Work out the finished part from the listing and answer in its coordinate system (mm). Face numbers are marked on the shaded views. Round coordinates to 2 decimals unless told otherwise and drop trailing zeros. Order: outer loops, then holes, each group sorted by start corner. A loop starts at its lowest first (then second) coordinate and runs counter-clockwise, first axis right, second up. Notation, with made-up numbers: (21, -16) - (27, -16) arc R19 ccw to (27, 10) - close; hole circle Ø1 at (-33, 22.25). An arc over 180 degrees is marked (long way). Answer in a Markdown table with one row per item.
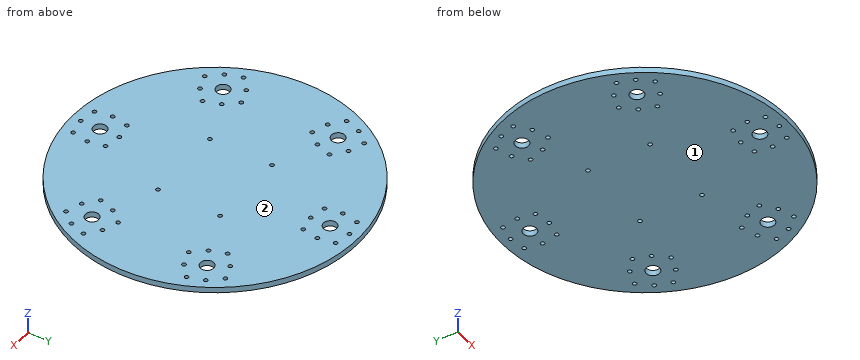
from build123d import *

# Parameters (mm, degrees)
SKETCH1_R           = 80
SKETCH1_R_2         = 1.1
SKETCH1_R_3         = 3.7
SKETCH1_R_4         = 1.11125
BOSS_EXTRUDE2_DEPTH = 3.175


with BuildPart() as part:
    # Sketch1 → Boss-Extrude2 (new body)
    with BuildSketch(Plane.XY):
        Circle(SKETCH1_R)
        with Locations((58.725568667, 44.315554285)):
            Circle(SKETCH1_R_2, mode=Mode.SUBTRACT)
        with Locations((67.741180127, 28.700057175)):
            Circle(SKETCH1_R_2, mode=Mode.SUBTRACT)
        with Locations((64.735398933, 37.375)):
            Circle(SKETCH1_R_2, mode=Mode.SUBTRACT)
        with Locations((50.050625842, 41.309773091)):
            Circle(SKETCH1_R_2, mode=Mode.SUBTRACT)
        with Locations((52.125683017, 19.684445715)):
            Circle(SKETCH1_R_2, mode=Mode.SUBTRACT)
        with Locations((43.110071557, 35.299942825)):
            Circle(SKETCH1_R_2, mode=Mode.SUBTRACT)
        with Locations((60.800625842, 22.690226909)):
            Circle(SKETCH1_R_2, mode=Mode.SUBTRACT)
        with Locations((46.115852752, 26.625)):
            Circle(SKETCH1_R_2, mode=Mode.SUBTRACT)
        with Locations((55.425625842, 32)):
            Circle(SKETCH1_R_3, mode=Mode.SUBTRACT)
        with Locations((-10.75, 64)):
            Circle(SKETCH1_R_2, mode=Mode.SUBTRACT)
        with Locations((-9.01561146, 73.01561146)):
            Circle(SKETCH1_R_2, mode=Mode.SUBTRACT)
        with Locations((9.01561146, 73.01561146)):
            Circle(SKETCH1_R_2, mode=Mode.SUBTRACT)
        with Locations((9.01561146, 54.98438854)):
            Circle(SKETCH1_R_2, mode=Mode.SUBTRACT)
        with Locations((-9.01561146, 54.98438854)):
            Circle(SKETCH1_R_2, mode=Mode.SUBTRACT)
        with Locations((0, 74.75)):
            Circle(SKETCH1_R_2, mode=Mode.SUBTRACT)
        with Locations((10.75, 64)):
            Circle(SKETCH1_R_2, mode=Mode.SUBTRACT)
        with Locations((0, 53.25)):
            Circle(SKETCH1_R_2, mode=Mode.SUBTRACT)
        with Locations((0, 64)):
            Circle(SKETCH1_R_3, mode=Mode.SUBTRACT)
        with Locations((67.741180127, -28.700057175)):
            Circle(SKETCH1_R_2, mode=Mode.SUBTRACT)
        with Locations((58.725568667, -44.315554285)):
            Circle(SKETCH1_R_2, mode=Mode.SUBTRACT)
        with Locations((64.735398933, -37.375)):
            Circle(SKETCH1_R_2, mode=Mode.SUBTRACT)
        with Locations((60.800625842, -22.690226909)):
            Circle(SKETCH1_R_2, mode=Mode.SUBTRACT)
        with Locations((43.110071557, -35.299942825)):
            Circle(SKETCH1_R_2, mode=Mode.SUBTRACT)
        with Locations((52.125683017, -19.684445715)):
            Circle(SKETCH1_R_2, mode=Mode.SUBTRACT)
        with Locations((50.050625842, -41.309773091)):
            Circle(SKETCH1_R_2, mode=Mode.SUBTRACT)
        with Locations((46.115852752, -26.625)):
            Circle(SKETCH1_R_2, mode=Mode.SUBTRACT)
        with Locations((55.425625842, -32)):
            Circle(SKETCH1_R_3, mode=Mode.SUBTRACT)
        with Locations((9.01561146, -73.01561146)):
            Circle(SKETCH1_R_2, mode=Mode.SUBTRACT)
        with Locations((-9.01561146, -73.01561146)):
            Circle(SKETCH1_R_2, mode=Mode.SUBTRACT)
        with Locations((0, -74.75)):
            Circle(SKETCH1_R_2, mode=Mode.SUBTRACT)
        with Locations((10.75, -64)):
            Circle(SKETCH1_R_2, mode=Mode.SUBTRACT)
        with Locations((-9.01561146, -54.98438854)):
            Circle(SKETCH1_R_2, mode=Mode.SUBTRACT)
        with Locations((9.01561146, -54.98438854)):
            Circle(SKETCH1_R_2, mode=Mode.SUBTRACT)
        with Locations((-10.75, -64)):
            Circle(SKETCH1_R_2, mode=Mode.SUBTRACT)
        with Locations((0, -53.25)):
            Circle(SKETCH1_R_2, mode=Mode.SUBTRACT)
        with Locations((0, -64)):
            Circle(SKETCH1_R_3, mode=Mode.SUBTRACT)
        with Locations((-58.725568667, -44.315554285)):
            Circle(SKETCH1_R_2, mode=Mode.SUBTRACT)
        with Locations((-67.741180127, -28.700057175)):
            Circle(SKETCH1_R_2, mode=Mode.SUBTRACT)
        with Locations((-64.735398933, -37.375)):
            Circle(SKETCH1_R_2, mode=Mode.SUBTRACT)
        with Locations((-50.050625842, -41.309773091)):
            Circle(SKETCH1_R_2, mode=Mode.SUBTRACT)
        with Locations((-52.125683017, -19.684445715)):
            Circle(SKETCH1_R_2, mode=Mode.SUBTRACT)
        with Locations((-43.110071557, -35.299942825)):
            Circle(SKETCH1_R_2, mode=Mode.SUBTRACT)
        with Locations((-60.800625842, -22.690226909)):
            Circle(SKETCH1_R_2, mode=Mode.SUBTRACT)
        with Locations((-46.115852752, -26.625)):
            Circle(SKETCH1_R_2, mode=Mode.SUBTRACT)
        with Locations((-55.425625842, -32)):
            Circle(SKETCH1_R_3, mode=Mode.SUBTRACT)
        with Locations((-67.741180127, 28.700057175)):
            Circle(SKETCH1_R_2, mode=Mode.SUBTRACT)
        with Locations((-58.725568667, 44.315554285)):
            Circle(SKETCH1_R_2, mode=Mode.SUBTRACT)
        with Locations((-64.735398933, 37.375)):
            Circle(SKETCH1_R_2, mode=Mode.SUBTRACT)
        with Locations((-60.800625842, 22.690226909)):
            Circle(SKETCH1_R_2, mode=Mode.SUBTRACT)
        with Locations((-43.110071557, 35.299942825)):
            Circle(SKETCH1_R_2, mode=Mode.SUBTRACT)
        with Locations((-52.125683017, 19.684445715)):
            Circle(SKETCH1_R_2, mode=Mode.SUBTRACT)
        with Locations((-50.050625842, 41.309773091)):
            Circle(SKETCH1_R_2, mode=Mode.SUBTRACT)
        with Locations((-46.115852752, 26.625)):
            Circle(SKETCH1_R_2, mode=Mode.SUBTRACT)
        with Locations((-55.425625842, 32)):
            Circle(SKETCH1_R_3, mode=Mode.SUBTRACT)
        with Locations((22.0345, 17.272)):
            Circle(SKETCH1_R_4, mode=Mode.SUBTRACT)
        with Locations((22.0345, -17.272)):
            Circle(SKETCH1_R_4, mode=Mode.SUBTRACT)
        with Locations((-21.9075, -17.272)):
            Circle(SKETCH1_R_4, mode=Mode.SUBTRACT)
        with Locations((-21.9075, 17.272)):
            Circle(SKETCH1_R_4, mode=Mode.SUBTRACT)
    extrude(amount=BOSS_EXTRUDE2_DEPTH)


solid = part.part
1) Find section C-C, the plane x = -27. Give the vertices of the cut face in (y, z) (3 decimals), then the cut area to 3 significant figures.
Filled in:
| item | result |
|---|---|
| outline | (-75.306, 0) - (75.306, 0) - (75.306, 3.175) - (-75.306, 3.175) - close |
| area | 478 mm^2 |
2) This flat-tipped pin is pushed along its axis until it touches: pin 1 (1 mm diameter, centred on y = -21, z = 2, fed in from +X). Where does it stop, or does it pass through?
Filled in:
| item | result |
|---|---|
| pin 1 | stops at x = 77.33 |
3) Find the intervals of material crossed by probe 1 along X at (y, z) = (54.5, 0.35); probe 2 along X at (y, z) = (-55.5, 0.7); probe 3 along Y at (x, z) = (-9.5, 0.9), in increasing order. Write a range as from..to.
Filled in:
| item | result |
|---|---|
| probe 1 | x = -58.56..-10, -8.03..8.03, 10..58.56 |
| probe 2 | x = -57.62..-9.99, -8.04..8.04, 9.99..57.62 |
| probe 3 | y = -79.43..-74, -72.03..-55.97, -54..54, 55.97..72.03, 74..79.43 |
4) The mould has two halves that part along Z. Classify the marked faces 1 and 2: released by +Z, released by -Z, zero draft, split by the parting line, or undercut.
Filled in:
| item | result |
|---|---|
| face 1 | released by -Z |
| face 2 | released by +Z |
5) Find section B-B, the plane z = 1.2. Give the number of separate pieces and of enclosed holes in the cut face, then the cut area to 3 significant figures.
Filled in:
| item | result |
|---|---|
| separate pieces | 1 |
| enclosed holes | 58 |
| area | 19,700 mm^2 |
6) Find section A-A, the plane y = -32. Give the vertices of the cut face in (x, z) (3 decimals).
Filled in:
| item | result |
|---|---|
| outline | (-73.321, 0) - (-59.126, 0) - (-59.126, 3.175) - (-73.321, 3.175) - close; (-51.726, 0) - (51.726, 0) - (51.726, 3.175) - (-51.726, 3.175) - close; (59.126, 0) - (73.321, 0) - (73.321, 3.175) - (59.126, 3.175) - close |
